```python
from build123d import *

# Parameters (mm, degrees)
SKETCH1_W           = 39
SKETCH1_H           = 9.5
BOSS_EXTRUDE1_DEPTH = 2.6
SKETCH3_W           = 2.6
SKETCH3_H           = 9.5
BOSS_EXTRUDE2_DEPTH = 3
SKETCH4_W           = 2
SKETCH4_H           = 6
CUT_EXTRUDE1_DEPTH  = 4


with BuildPart() as part:
    # Sketch1 → Boss-Extrude1 (new body)
    with BuildSketch(Plane.XY):
        with Locations((-13.141843972, 13.308510638)):
            Rectangle(SKETCH1_W, SKETCH1_H)
    extrude(amount=BOSS_EXTRUDE1_DEPTH)

    # Sketch3 → Boss-Extrude2 (add)
    with BuildSketch(Plane.XY.offset(2.6)):
        with Locations((-31.341843972, 13.308510638)):
            Rectangle(SKETCH3_W, SKETCH3_H)
    extrude(amount=BOSS_EXTRUDE2_DEPTH)

    # Sketch4 → Cut-Extrude1 (cut)
    with BuildSketch(Plane(origin=(0, 0, 0), x_dir=(-1, 0, 0), z_dir=(0, 0, -1))):
        with Locations((-3.358156028, 13.308510638)):
            Rectangle(SKETCH4_W, SKETCH4_H)
    extrude(amount=-CUT_EXTRUDE1_DEPTH, mode=Mode.SUBTRACT)


solid = part.part
```
The model under review builds one solid part; all positions refer to its coordinate system, in mm. A direction names the side the tool comes from. Round coordinates to 2 decimals unless told otherwise and drop trailing zeros. Write each loop counter-clockwise with the first axis right and the second up, starting at its lowest first coordinate (ties: lowest second). Pieces come first, ordered by that corner, then holes. Notation, with made-up numbers: (-36, 70) -> (-4, 70) arc R24 cw to (-4, 94) -> close; hole circle Ø5 at (-37.75, 24.25). An arc over 180 degrees is marked (long way). Use CSV: the item, a comma, the result in double quotes.
Q1. For faces 5 (the flat face through (-13, 13, 0)), 6 (the flat face through (-30.042, 13, 4)), 7 (the flat face through (2.358, 13, 1)), list the 3-axis set-ups (+Z, -Z, +X, -X, +Y, -Y) from which the entire face can be reached by the end or side of a thin tool; tool diameter is ignored.
Checks:
face 5,"-Z, +X, -X, +Y, -Y"
face 6,"+Z, +X, +Y, -Y"
face 7,"+Z, -Z"
Q2. Consider section A-A (y = 13.75). Give the boundary of the cut face in (x, z), then the cut area to 3 significant figures.
Checks:
outline,"(-32.64, 0) -> (2.36, 0) -> (2.36, 2.6) -> (-30.04, 2.6) -> (-30.04, 5.6) -> (-32.64, 5.6) -> close; (4.36, 0) -> (6.36, 0) -> (6.36, 2.6) -> (4.36, 2.6) -> close"
area,"104 mm²"
Q3. Consider section D-D (z = 2.95). Give the boundary of the cut face in (x, y).
Checks:
outline,"(-32.64, 8.56) -> (-30.04, 8.56) -> (-30.04, 18.06) -> (-32.64, 18.06) -> close"
Q4. Consider section C-C (x = 4). Give the boundary of the cut face in (y, z).
Checks:
outline,"(8.56, 0) -> (10.31, 0) -> (10.31, 2.6) -> (8.56, 2.6) -> close; (16.31, 0) -> (18.06, 0) -> (18.06, 2.6) -> (16.31, 2.6) -> close"
Q5. Consider section B-B (z = 0.4). Give the boundary of the cut face in (x, y).
Checks:
outline,"(-32.64, 8.56) -> (6.36, 8.56) -> (6.36, 18.06) -> (-32.64, 18.06) -> close; hole (2.36, 10.31) -> (4.36, 10.31) -> (4.36, 16.31) -> (2.36, 16.31) -> close"
Q6. Mouldability with a two-part tool opening along X and no side actions: class faces 1 (the flat face through (-13, 18.059, 2)), 2 (the flat face through (3, 16.309, 1)), 3 (the flat face through (-32.642, 13, 3)), 4 (the flat face through (4.358, 13, 1)) as released by +X, released by -X, zero draft, split by the parting line, or undercut.
Checks:
face 1,"zero draft"
face 2,"undercut"
face 3,"released by -X"
face 4,"undercut"
Q7. For pin 1 Ø3 at (x, y) = (-13.5, 15) entering from +Z; pin 2 Ø0.9 at (y, z) = (12.5, 3.5) entering from +X, all flat-tipped, find the tip position at first contact; note any pin that passes through.
Checks:
pin 1,"z = 2.6"
pin 2,"x = -30.04"
Q8. To check wall thickness, follow probe 1 along X at (y, z) = (14.75, 0.55); probe 2 along X at (y, z) = (14.5, 2.95); probe 3 along Z at (x, y) = (2.5, 17.5). State the ranges of each line that lie inside material, in increasing order. Write a range as [from, to].
Checks:
probe 1,"[-32.64, 2.36], [4.36, 6.36]"
probe 2,"[-32.64, -30.04]"
probe 3,"[0, 2.6]"
